The model under review builds one solid part; all positions refer to its coordinate system, in mm. Face numbers are marked on the shaded views. A direction names the side the tool comes from. Give positions to 0.01 mm unless a question says otherwise; leave off trailing zeros. Order: outer loops, then holes, each group sorted by start corner. A loop starts at its lowest first (then second) coordinate and runs counter-clockwise, first axis right, second up. Notation, with made-up numbers: (-19.75, -24) - (24.25, -24) arc R15 cw to (24.25, -15) - close; hole circle Ø5 at (82, 85.5). An arc over 180 degrees is marked (long way). Use CSV: the item, a comma, the result in double quotes.
```python
from build123d import *

# Parameters (mm, degrees)
F1_DEPTH = 317.5
F2_T     = -3.175
F4_DEPTH = 1.5875
F5_W     = 508
F5_H     = 889
F6_DEPTH = 4.9404231503


with BuildPart() as f1:
    # F0 (on Right) → F1 (new body, symmetric)
    with BuildSketch(Plane.YZ):
        Polygon((-340.995, 0), (0, 0), (0, 1454.5287787333), (-340.995, 1168.4), align=None)
    extrude(amount=F1_DEPTH, both=True)

    # F2
    f2_openings = [f1.faces().sort_by_distance(p)[0] for p in [
        (0, 0, 727.264389),
    ]]
    offset(amount=F2_T, openings=f2_openings)

    # F3 (on Front) → F4 (join, symmetric)
    with BuildSketch(Plane.XZ):
        Polygon((-273.1135, 247.904), (273.1135, 247.904), (273.1135, 0), (317.5, 0), (317.5, 247.904), (317.5, 1206.6247787333), (317.5, 1454.5287787333), (273.1135, 1454.5287787333), (273.1135, 1206.6247787333), (-273.1135, 1206.6247787333), (-273.1135, 1454.5287787333), (-317.5, 1454.5287787333), (-317.5, 1206.6247787333), (-317.5, 247.904), (-317.5, 0), (-273.1135, 0), align=None)
    extrude(amount=F4_DEPTH, both=True)

    # F5 (on face) → F6 (cut, through all)
    with BuildSketch(Plane.XZ.offset(340.995)):
        with Locations((0, 723.9)):
            Rectangle(F5_W, F5_H)
    extrude(amount=-F6_DEPTH, mode=Mode.SUBTRACT)


solid = f1.part
```
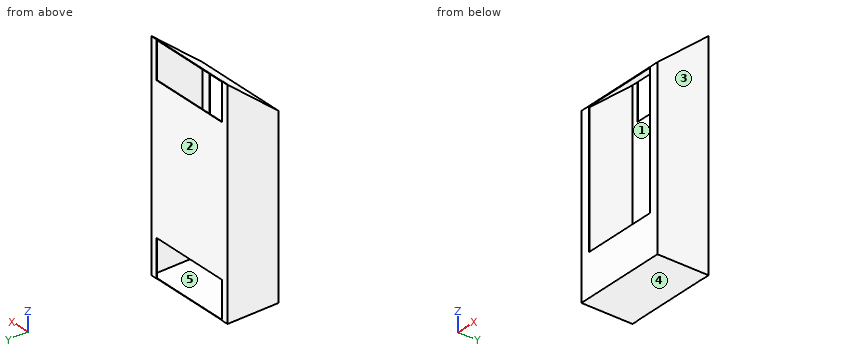
Item 1: Wall thickness on L1, parallel to X at y = -318, z = 1073 (3 decimals); L2, parallel to Y at x = 51, z = 1089.5; L3, parallel to Z at x = 188, y = -69 (3 decimals): over which ranges is each line inside the solid? List them lowest first.
Results list:
L1,"x = -317.5 to -314.325, 314.325 to 317.5"
L2,"y = -1.59 to 1.59"
L3,"z = 0 to 3.175, 1392.486 to 1396.631"
Item 2: Mouldability with a two-part tool opening along X and no side actions: class the marked faces 1, 2 and 3 as pulls with the +X half, pulls with the -X half, needs draft (parallel to the pull), parting line crosses it, or undercut.
Results list:
face 1,"undercut"
face 2,"needs draft"
face 3,"pulls with the +X half"
Item 3: Take a section at A-A, the plane x = -171. Give the boundary of the cut face in (y, z) (1 decimal), and give its area (3 significant figures).
Results list:
outline,"(-341, 0) - (0, 0) - (0, 3.2) - (-337.8, 3.2) - (-337.8, 279.4) - (-341, 279.4) - close; (-341, 1168.4) - (-336.1, 1168.4) - (0, 1450.4) - (0, 1454.5) - close; (-1.6, 247.9) - (1.6, 247.9) - (1.6, 1206.6) - (-1.6, 1206.6) - close"
area,"6,410 mm2"
Item 4: Take a section at C-C, the plane z = 1089. Give the boundary of the cut face in (x, y) (1 decimal), and give its area (3 significant figures).
Results list:
outline,"(-317.5, -341) - (-254, -341) - (-254, -337.8) - (-314.3, -337.8) - (-314.3, -1.6) - (314.3, -1.6) - (314.3, -337.8) - (254, -337.8) - (254, -341) - (317.5, -341) - (317.5, 1.6) - (-317.5, 1.6) - close"
area,"4,550 mm2"
Item 5: Tool access review of the marked faces 4 and 5: name each direction out of +Z, -Z, +X, -X, +Y, -Y from which nothing blocks a thin tool from reaching the whole face with its end or side.
Results list:
face 4,"-Z, +X, -X, +Y, -Y"
face 5,"none"
Item 6: Take a section at B-B, the plane y = -112. Give the boundary of the cut face in (x, z) (3 decimals), and give its area (3 significant figures).
Results list:
outline,"(-317.5, 0) - (317.5, 0) - (317.5, 1360.55) - (-317.5, 1360.55) - close; hole (-314.325, 3.175) - (314.325, 3.175) - (314.325, 1356.405) - (-314.325, 1356.405) - close"
area,"13,200 mm2"
Item 7: Clearance check with flat-ended pins moving along their axes: pin 1 (3 mm diameter, centred on x = 175.5, z = 1216, fed in from -Y); pin 2 (3 mm diameter, centred on x = 225, z = 465.5, fed in from -Y); pin 3 (2 mm diameter, centred on x = 69, z = 1453, fed in from +Y). State where each tip first meets the part, or that it passes through.
Results list:
pin 1,"stops at y = -286.06"
pin 2,"stops at y = -1.59"
pin 3,"stops at y = 0"
Item 8: Take a section at D-D, the plane y = -28.5. Give the boundary of the cut face in (x, z) (3 decimals), and give its area (3 significant figures).
Results list:
outline,"(-317.5, 0) - (317.5, 0) - (317.5, 1430.614) - (-317.5, 1430.614) - close; hole (-314.325, 3.175) - (314.325, 3.175) - (314.325, 1426.47) - (-314.325, 1426.47) - close"
area,"13,700 mm2"
